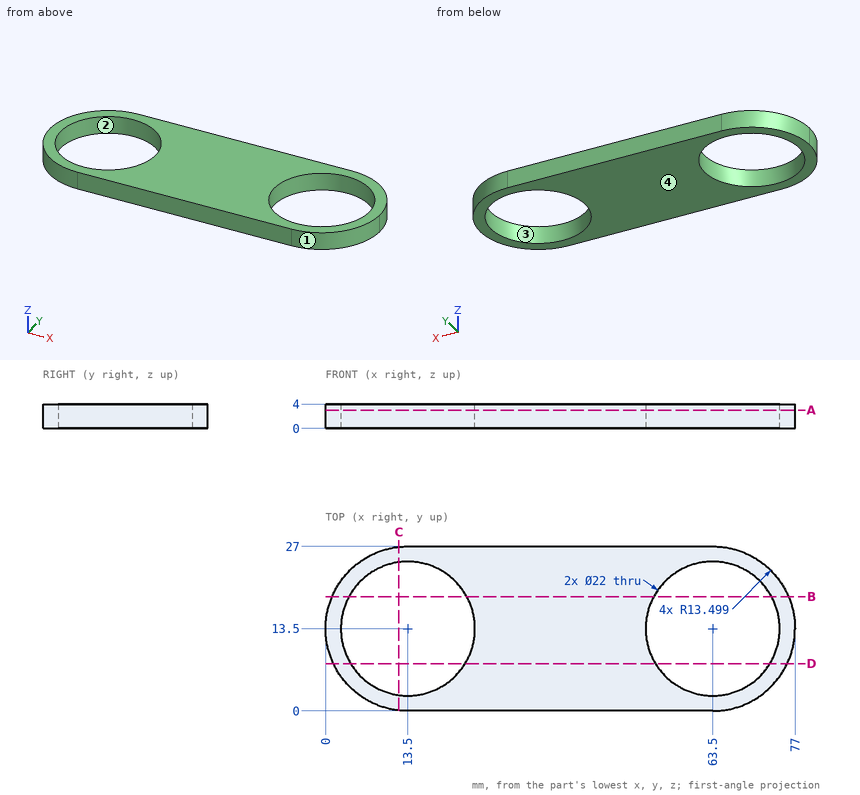
The figure shows three views and two pictorial views of one solid part (mm, origin at its lowest corner). Answer the questions. Round coordinates to 2 decimals unless told otherwise and drop trailing zeros. Order: outer loops, then holes, each group sorted by start corner. A loop starts at its lowest first (then second) coordinate and runs counter-clockwise, first axis right, second up. Notation, with made-up numbers: (86.25, 79.5) -> (120.25, 79.5) arc R27 cw to (120.25, 108.5) -> close; hole circle Ø1 at (3.25, 80.5). An arc over 180 degrees is marked (long way). One line per item, written item: value.
Item 1: Straight lines are drawn through the part: L1, parallel to Y at x = 63.5, z = 2.85; L2, parallel to X at y = 8, z = 2.5 (1 decimal); L3, parallel to X at y = 19.5, z = 1.75 (1 decimal). For each, find the intervals that lie inside material, in ascending order.
Taken from the geometry:
L1: y = 0 to 2.5, 24.5 to 27
L2: x = 1.2 to 4, 23 to 54, 73 to 75.8
L3: x = 1.4 to 4.3, 22.7 to 54.3, 72.7 to 75.6
Item 2: Find section B-B, the plane y = 18.75. Give the vertices of the cut face in (x, z).
Taken from the geometry:
outline: (1.06, 0) -> (3.83, 0) -> (3.83, 4) -> (1.06, 4) -> close; (23.17, 0) -> (53.83, 0) -> (53.83, 4) -> (23.17, 4) -> close; (73.17, 0) -> (75.94, 0) -> (75.94, 4) -> (73.17, 4) -> close
Item 3: Find section D-D, the plane y = 7.75. Give the vertices of the cut face in (x, z) (1 decimal), then the cut area to 3 significant figures.
Taken from the geometry:
outline: (1.3, 0) -> (4.1, 0) -> (4.1, 4) -> (1.3, 4) -> close; (22.9, 0) -> (54.1, 0) -> (54.1, 4) -> (22.9, 4) -> close; (72.9, 0) -> (75.7, 0) -> (75.7, 4) -> (72.9, 4) -> close
area: 148 mm2
Item 4: Find section A-A, the plane z = 3. State how many separate pieces and enclosed holes the cut face has, then the cut area to 3 significant figures.
Taken from the geometry:
separate pieces: 1
enclosed holes: 2
area: 1,160 mm2
Item 5: Given P1, Ø2, axis at x = 37.5, z = 2, coming from the -Y side, flat-ended and moving along its own axis, determine where the tip first touches the part or whether it passes through.
Taken from the geometry:
P1: stops at y = 0
Item 6: For a pull along Y with two mould halves and no side action, classify the marked faces 1, 2, 3 and 4 as released by +Y, released by -Y, zero draft, split by the parting line, or undercut.
Taken from the geometry:
face 1: released by -Y
face 2: undercut
face 3: undercut
face 4: zero draft
Item 7: Find section C-C, the plane x = 12. Give the vertices of the cut face in (y, z).
Taken from the geometry:
outline: (0.08, 0) -> (2.6, 0) -> (2.6, 4) -> (0.08, 4) -> close; (24.4, 0) -> (26.92, 0) -> (26.92, 4) -> (24.4, 4) -> close
